from build123d import *

# Parameters (mm, degrees)
F0_W     = 3.2
F0_H     = 3.2
F1_DEPTH = 8
F3_DEPTH = 25


with BuildPart() as f1:
    # F0 (on Top) → F1 (new body)
    with BuildSketch(Plane.XY):
        with Locations((1.6, 1.6)):
            Rectangle(F0_W, F0_H)
    extrude(amount=F1_DEPTH)

    # F2 (on face) → F3 (cut)
    with BuildSketch(Plane.XY.offset(8)):
        with BuildLine():
            Line((2.3035712473, 0.8964287527), (0.8964287527, 2.3035712473))
            ThreePointArc((0.8964287527, 2.3035712473), (0.8964287527, 0.8964287527), (2.3035712473, 0.8964287527))
        make_face()
        with BuildLine():
            ThreePointArc((2.595, 1.6), (1.9807700152, 2.5192601348), (0.8964287527, 2.3035712473))
            Line((0.8964287527, 2.3035712473), (2.3035712473, 0.8964287527))
            ThreePointArc((2.3035712473, 0.8964287527), (2.5192601348, 1.2192299848), (2.595, 1.6))
        make_face()
    extrude(amount=-F3_DEPTH, mode=Mode.SUBTRACT)


solid = f1.part
Input: part model. Units: mm. Frame: model coordinates. Give positions to 0.01 mm unless a question says otherwise; leave off trailing zeros. Order: outer loops, then holes, each group sorted by start corner. A loop starts at its lowest first (then second) coordinate and runs counter-clockwise, first axis right, second up.
Q1. Section A-A on x = 1.6. Output: boundary loops of the cut face in (y, z) (3 decimals).
Checked values:
outline: (0, 0) - (0.605, 0) - (0.605, 8) - (0, 8) - close; (2.595, 0) - (3.2, 0) - (3.2, 8) - (2.595, 8) - close
Q2. Section C-C on z = 2. Output: boundary loops of the cut face in (x, y) (3 decimals), and give its area (3 significant figures).
Checked values:
outline: (0, 0) - (3.2, 0) - (3.2, 3.2) - (0, 3.2) - close; hole circle Ø1.99 at (1.6, 1.6)
area: 7.13 mm2
Q3. Section B-B on y = 2.05. Output: boundary loops of the cut face in (x, z).
Checked values:
outline: (0, 0) - (0.71, 0) - (0.71, 8) - (0, 8) - close; (2.49, 0) - (3.2, 0) - (3.2, 8) - (2.49, 8) - close
Q4. Ray query, probe 1 along Y at (x, z) = (1.55, 7.5); probe 2 along X at (y, z) = (1.15, 3); probe 3 along Y at (x, z) = (0.9, 0.5). Return the intervals inside material, ascending.
Checked values:
probe 1: y = 0 to 0.61, 2.59 to 3.2
probe 2: x = 0 to 0.71, 2.49 to 3.2
probe 3: y = 0 to 0.89, 2.31 to 3.2
